Source: CAD feature listing. Evaluate the final solid. Frame: model axes, mm. Face numbers are marked on the shaded views. A direction names the side the tool comes from. Round coordinates to 2 decimals unless told otherwise and drop trailing zeros. Order: outer loops, then holes, each group sorted by start corner. A loop starts at its lowest first (then second) coordinate and runs counter-clockwise, first axis right, second up. Notation, with made-up numbers: (-23, -37.5) -> (16, -37.5) arc R17 ccw to (16, -11.5) -> close; hole circle Ø6 at (-6.5, 17). An arc over 180 degrees is marked (long way). Answer as CSV lines item,"result".
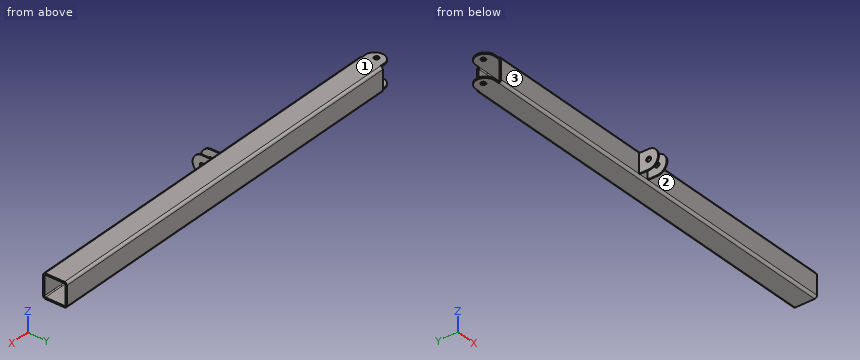
from build123d import *

# Parameters (mm, degrees)
EXTRUDE_THIN1_DEPTH      = 820
SKETCH3_R                = 5
BOSS_EXTRUDE2_DEPTH      = 3
BOSS_EXTRUDE3_START      = -47
SKETCH3_3_R              = 5
BOSS_EXTRUDE3_DEPTH      = 3
BOSS_EXTRUDE4_DEPTH      = 40
BOSS_EXTRUDE4_DEPTH_BACK = 10
FILLET1_R                = 20
SKETCH7_R                = 5
CUT_EXTRUDE3_DEPTH       = 444.504548848


with BuildPart() as part:
    # Sketch1 → Extrude-Thin1 (new body)
    with BuildSketch(Plane(origin=(0, 0, 0), x_dir=(0, 0, -1), z_dir=(1, 0, 0))):
        with BuildLine():
            Line((-25, 20), (-25, -20))
            ThreePointArc((-25, -20), (-23.535533906, -23.535533906), (-20, -25))
            Line((-20, -25), (20, -25))
            ThreePointArc((20, -25), (23.535533906, -23.535533906), (25, -20))
            Line((25, -20), (25, 20))
            ThreePointArc((25, 20), (23.535533906, 23.535533906), (20, 25))
            Line((20, 25), (-20, 25))
            ThreePointArc((-20, 25), (-23.535533906, 23.535533906), (-25, 20))
        make_face()
        with BuildLine():
            Line((-22, 20), (-22, -20))
            ThreePointArc((-22, -20), (-21.414213562, -21.414213562), (-20, -22))
            Line((-20, -22), (20, -22))
            ThreePointArc((20, -22), (21.414213562, -21.414213562), (22, -20))
            Line((22, -20), (22, 20))
            ThreePointArc((22, 20), (21.414213562, 21.414213562), (20, 22))
            Line((20, 22), (-20, 22))
            ThreePointArc((-20, 22), (-21.414213562, 21.414213562), (-22, 20))
        make_face(mode=Mode.SUBTRACT)
    extrude(amount=EXTRUDE_THIN1_DEPTH)

    # Sketch3 → Boss-Extrude2 (add)
    with BuildSketch(Plane(origin=(0, 0, -25), x_dir=(-1, 0, 0), z_dir=(0, 0, -1))):
        with BuildLine():
            Line((0, 20), (10, 20))
            ThreePointArc((10, 20), (30, 0), (10, -20))
            Line((10, -20), (0, -20))
            Line((0, -20), (0, 20))
        make_face()
        with Locations((15, 0)):
            Circle(SKETCH3_R, mode=Mode.SUBTRACT)
    extrude(amount=-BOSS_EXTRUDE2_DEPTH)

    # Sketch3<3> → Boss-Extrude3 (add)
    with BuildSketch(Plane(origin=(0, 0, -25), x_dir=(-1, 0, 0), z_dir=(0, 0, -1)).offset(BOSS_EXTRUDE3_START)):
        with BuildLine():
            Line((0, 20), (10, 20))
            ThreePointArc((10, 20), (30, 0), (10, -20))
            Line((10, -20), (0, -20))
            Line((0, -20), (0, 20))
        make_face()
        with Locations((15, 0)):
            Circle(SKETCH3_3_R, mode=Mode.SUBTRACT)
    extrude(amount=-BOSS_EXTRUDE3_DEPTH)

    # Sketch5 → Boss-Extrude4 (add, two sides: drawn at the far end of the back side and taken through both)
    with BuildSketch(Plane.XZ.offset(25).offset(-BOSS_EXTRUDE4_DEPTH_BACK)):
        Polygon((358, -19.999999922), (358.002493701, 20), (360, 20), (360, -20), align=None)
        Polygon((380, 20), (381.997506299, 20), (382, -19.999999922), (380, -20), align=None)
    extrude(amount=BOSS_EXTRUDE4_DEPTH + BOSS_EXTRUDE4_DEPTH_BACK)

    # Fillet1
    fillet1_edges = [part.edges().sort_by_distance(p)[0] for p in [
        (380.99875315, -65, 20),
        (381, -65, -19.999999961),
        (359.00124685, -65, 20),
        (359, -65, -19.999999961),
    ]]
    fillet(fillet1_edges, radius=FILLET1_R - 0.0001)  # a hair under: the kernel refuses the full size

    # Sketch7 → Cut-Extrude3 (cut, through all)
    with BuildSketch(Plane(origin=(381.998751665, 0, 0.023814765), x_dir=(6.234251963554982e-05, 0, -0.9999999980567051), z_dir=(0.9999999980567051, 0, 6.234251963554982e-05))):
        with Locations((0.023814765, -45)):
            Circle(SKETCH7_R)
    extrude(amount=-CUT_EXTRUDE3_DEPTH, mode=Mode.SUBTRACT)


solid = part.part
1. Pin query (flat end, axial travel): pin 1 (6 mm diameter, centred on x = 420, z = -3, fed in from -Y); pin 2 (6 mm diameter, centred on x = -15, y = 0, fed in from +Z); pin 3 (2 mm diameter, centred on x = 359, y = -33.5, fed in from -Z); pin 4 (0.9 mm diameter, centred on x = -3.5, z = 23.5, fed in from -Y). Return the tip coordinate at first contact, or that it passes through.
Results below:
pin 1,"y = -25"
pin 2,"through"
pin 3,"z = -20"
pin 4,"y = -20"
2. Reachability of the marked faces 1, 2 and 3 from +Z, -Z, +X, -X, +Y, -Y: full face, straight path, thin tool, end or side. Return the list, or none.
Results below:
face 1,"+Z, +X, -X, +Y, -Y"
face 2,"+Z, -Z, +X, -Y"
face 3,"+Z, -Z, -X, -Y"
3. Section query A-A on x = 152.5. Return loops of the section in (y, z).
Results below:
outline,"(-25, -20) arc R5 ccw to (-20, -25) -> (20, -25) arc R5 ccw to (25, -20) -> (25, 20) arc R5 ccw to (20, 25) -> (-20, 25) arc R5 ccw to (-25, 20) -> close; hole (-22, -20) arc R2 ccw to (-20, -22) -> (20, -22) arc R2 ccw to (22, -20) -> (22, 20) arc R2 ccw to (20, 22) -> (-20, 22) arc R2 ccw to (-22, 20) -> close"
4. Line query: L1, parallel to Y at x = 381, z = 0; L2, parallel to Z at x = 744, y = 2; L3, parallel to X at y = -32, z = 4.5. Output: solid intervals per line, ascending. Write a range as [from, to].
Results below:
L1,"[-65, -50], [-40, -15], [22, 25]"
L2,"[-25, -22], [22, 25]"
L3,"[358, 360], [380, 382]"
